```python
from build123d import *
from OCP.BRepFilletAPI import BRepFilletAPI_MakeChamfer

# Parameters (mm, degrees)
SKETCH1_W               = 29.5
SKETCH1_H               = 29.5
BOSS_EXTRUDE1_DEPTH     = 10
SKETCH2_R               = 12.5
CUT_EXTRUDE1_DEPTH      = 5
CHAMFER1_SIZE           = 22.860104606
CHAMFER1_SIZE_2         = 2
CHAMFER2_SIZE           = 4
CHAMFER2_SIZE2          = 4.030734246
SKETCH5_R               = 8
CUT_EXTRUDE2_DEPTH      = 10
BOSS_EXTRUDE2_START     = -1
BOSS_EXTRUDE2_DEPTH     = 1
MIRROR2_START           = -1
MIRROR2_COPY_1_DEPTH    = 1
CUT_EXTRUDE3_DEPTH      = 43.277768842
CUT_EXTRUDE3_DEPTH_BACK = 43.277768842
SKETCH7_R               = 1.125
SKETCH8_R               = 0.635
CUT_EXTRUDE4_DEPTH      = 43.501879232
SKETCH10_R              = 0.915
CUT_EXTRUDE5_DEPTH      = 2
SKETCH11_OUTSIDE_W      = 39.354
SKETCH11_OUTSIDE_H      = 39.324
SKETCH11_OUTSIDE_R      = 19
CUT_EXTRUDE6_DEPTH      = 43.501879232
SKETCH12_R              = 2
CUT_EXTRUDE7_DEPTH      = 9
SKETCH13_W              = 11
SKETCH13_H              = 30.855989766
CUT_EXTRUDE8_DEPTH      = 7


with BuildPart() as part:
    # Sketch1 → Boss-Extrude1 (new body)
    with BuildSketch(Plane(origin=(0, 0, 0), x_dir=(1, 0, 0), z_dir=(0, 1, 0))):
        with Locations((14.75, 14.75)):
            Rectangle(SKETCH1_W, SKETCH1_H)
    extrude(amount=BOSS_EXTRUDE1_DEPTH)

    # Sketch2 → Cut-Extrude1 (cut)
    with BuildSketch(Plane(origin=(0, 10, 0), x_dir=(1, 0, 0), z_dir=(0, 1, 0))):
        with Locations(Location((14.75, 14.75, 0), (0, 0, 270))):
            Circle(SKETCH2_R)
    extrude(amount=-CUT_EXTRUDE1_DEPTH, mode=Mode.SUBTRACT)

    # Chamfer1
    # the kernel refuses this chamfer: 22.860104606, 2 mm, written as the material it takes off along each edge
    with BuildSketch(Plane(origin=(-59.427907001, 0, 0), x_dir=(0, 1, 0), z_dir=(1, 0, 0)), Plane(origin=(29.5, 0, 59.427907001), x_dir=(0, 1, 0), z_dir=(0, 0, -1)), Plane(origin=(0, 0, -88.927907001), x_dir=(0, 1, 0), z_dir=(0, 0, 1))) as chamfer1_piece_1:
        Polygon((CHAMFER1_SIZE, 0), (0, -CHAMFER1_SIZE_2), (0, 0), align=None)
    extrude(amount=148.355814002, mode=Mode.SUBTRACT)
    with BuildSketch(Plane(origin=(88.927907001, 0, -29.5), x_dir=(0, 0, 1), z_dir=(-1, 0, 0))) as chamfer1_piece_2:
        Polygon((CHAMFER1_SIZE_2, 0), (0, CHAMFER1_SIZE), (0, 0), align=None)
    extrude(amount=148.355814002, mode=Mode.SUBTRACT)

    # Chamfer2: one chamfer whose edges measure the first distance from different faces: ONE call of the kernel's chamfer builder (chamfer() names one face for all edges)
    chamfer2_edges_1 = [part.edges().sort_by_distance(p)[0] for p in [
        (1.562556682, 5, -27.937443318),
        (27.937443318, 5, -27.937443318),
    ]]
    chamfer2_side_1 = [part.faces().sort_by_distance(p)[0] for p in [
        (14.75, 5.055285333, -27.942280158),
    ]]
    chamfer2_edges_2 = [part.edges().sort_by_distance(p)[0] for p in [
        (1.562556682, 5, -1.562556682),
    ]]
    chamfer2_side_2 = [part.faces().sort_by_distance(p)[0] for p in [
        (1.557719842, 5.055285333, -14.75),
    ]]
    chamfer2_edges_3 = [part.edges().sort_by_distance(p)[0] for p in [
        (27.937443318, 5, -1.562556682),
    ]]
    chamfer2_side_3 = [part.faces().sort_by_distance(p)[0] for p in [
        (27.942280158, 5.055285333, -14.75),
    ]]
    chamfer2 = BRepFilletAPI_MakeChamfer(part.part.solid().wrapped)
    for e in chamfer2_edges_1:
        chamfer2.Add(CHAMFER2_SIZE, CHAMFER2_SIZE2, e.wrapped, chamfer2_side_1[0].wrapped)  # the first distance lies on this face
    for e in chamfer2_edges_2:
        chamfer2.Add(CHAMFER2_SIZE, CHAMFER2_SIZE2, e.wrapped, chamfer2_side_2[0].wrapped)  # the first distance lies on this face
    for e in chamfer2_edges_3:
        chamfer2.Add(CHAMFER2_SIZE, CHAMFER2_SIZE2, e.wrapped, chamfer2_side_3[0].wrapped)  # the first distance lies on this face
    add(Compound.cast(chamfer2.Shape()), mode=Mode.REPLACE)

    # Sketch5 → Cut-Extrude2 (cut)
    with BuildSketch(Plane.XZ):
        with Locations(Location((14.75, -14.734574622, 0), (0, 0, 270))):
            Circle(SKETCH5_R)
    extrude(amount=-CUT_EXTRUDE2_DEPTH, mode=Mode.SUBTRACT)

    # Boss-Extrude2: read off the stored shape, not the designer's step
    # Boss-Extrude2 outline → Boss-Extrude2 (add)
    with BuildSketch(Plane(origin=(0, 10, 0), x_dir=(1, 0, 0), z_dir=(0, 1, 0)).offset(BOSS_EXTRUDE2_START)):
        with BuildLine():
            Line((1.125113365, 5.14027687), (5.171127626, 1.125113365))
            Line((5.171127626, 1.125113365), (24.328872374, 1.125113365))
            Line((24.328872374, 1.125113365), (28.374886635, 5.14027687))
            Line((28.374886635, 5.14027687), (28.374886635, 24.328872374))
            Line((28.374886635, 24.328872374), (24.35972313, 28.374886635))
            Line((24.35972313, 28.374886635), (5.14027687, 28.374886635))
            ThreePointArc((5.14027687, 28.374886635), (1.109687987, 28.359461258), (1.125113365, 24.328872374))
            Line((1.125113365, 24.328872374), (1.125113365, 5.14027687))
        make_face()
        Polygon((24.272234466, 28.287397972), (28.287397972, 24.241383711), (28.287397972, 5.227765534), (24.241383711, 1.212602028), (5.258616289, 1.212602028), (1.212602028, 5.227765534), (1.212602028, 24.241383711), (5.227765534, 28.287397972), align=None, mode=Mode.SUBTRACT)
    boss_extrude2 = extrude(amount=BOSS_EXTRUDE2_DEPTH)

    # Mirror1: Boss-Extrude2 across plane
    add(boss_extrude2.mirror(Plane(origin=(14.75, 0, 0), x_dir=(0, 0, 1), z_dir=(1, 0, 0))))

    # Mirror2: Boss-Extrude2 across plane
    add(boss_extrude2.mirror(Plane.XY.offset(-14.75)))

    # Mirror2 copy 1 sketch → Mirror2 copy 1 (add)
    with BuildSketch(Plane(origin=(29.5, 10, -29.5), x_dir=(-1, 0, 0), z_dir=(0, 1, 0)).offset(MIRROR2_START)):
        with BuildLine():
            Line((1.125113365, 5.14027687), (5.171127626, 1.125113365))
            Line((5.171127626, 1.125113365), (24.328872374, 1.125113365))
            Line((24.328872374, 1.125113365), (28.374886635, 5.14027687))
            Line((28.374886635, 5.14027687), (28.374886635, 24.328872374))
            Line((28.374886635, 24.328872374), (24.35972313, 28.374886635))
            Line((24.35972313, 28.374886635), (5.14027687, 28.374886635))
            ThreePointArc((5.14027687, 28.374886635), (1.109687987, 28.359461258), (1.125113365, 24.328872374))
            Line((1.125113365, 24.328872374), (1.125113365, 5.14027687))
        make_face()
        Polygon((24.272234466, 28.287397972), (28.287397972, 24.241383711), (28.287397972, 5.227765534), (24.241383711, 1.212602028), (5.258616289, 1.212602028), (1.212602028, 5.227765534), (1.212602028, 24.241383711), (5.227765534, 28.287397972), align=None, mode=Mode.SUBTRACT)
    extrude(amount=MIRROR2_COPY_1_DEPTH)

    # Sketch7 → Cut-Extrude3 (cut, two sides: drawn at the far end of the back side and taken through both)
    with BuildSketch(Plane.XZ.offset(-9).offset(-CUT_EXTRUDE3_DEPTH_BACK)):
        with Locations(Location((3.132695117, -3.148120495, 0), (0, 0, 270))):
            Circle(SKETCH7_R)
        with Locations(Location((26.367304883, -3.148120495, 0), (0, 0, 308.909428046))):
            Circle(SKETCH7_R)
        with Locations(Location((26.367304883, -26.351879505, 0), (0, 0, 270))):
            Circle(SKETCH7_R)
        with Locations(Location((3.132695117, -26.351879505, 0), (0, 0, 270))):
            Circle(SKETCH7_R)
    extrude(amount=CUT_EXTRUDE3_DEPTH + CUT_EXTRUDE3_DEPTH_BACK, mode=Mode.SUBTRACT)

    # Sketch8 → Cut-Extrude4 (cut, through all)
    with BuildSketch(Plane.XZ):
        with Locations(Location((7.375113365, -5.625113365, 0), (0, 0, 270))):
            Circle(SKETCH8_R)
        with Locations(Location((7.375113365, -23.874886635, 0), (0, 0, 270))):
            Circle(SKETCH8_R)
        with Locations(Location((4.625113365, -14.75, 0), (0, 0, 270))):
            Circle(SKETCH8_R)
        with Locations(Location((22.124886635, -23.874886635, 0), (0, 0, 90))):
            Circle(SKETCH8_R)
        with Locations(Location((24.874886635, -14.75, 0), (0, 0, 90))):
            Circle(SKETCH8_R)
        with Locations(Location((22.124886635, -5.625113365, 0), (0, 0, 90))):
            Circle(SKETCH8_R)
        with Locations(Location((5.770249527, -10.25, 0), (0, 0, 270))):
            Circle(SKETCH8_R)
        with Locations(Location((5.770249527, -19.25, 0), (0, 0, 90))):
            Circle(SKETCH8_R)
        with Locations(Location((23.729750473, -10.25, 0), (0, 0, 90))):
            Circle(SKETCH8_R)
        with Locations(Location((23.729750473, -19.25, 0), (0, 0, 270))):
            Circle(SKETCH8_R)
    extrude(amount=-CUT_EXTRUDE4_DEPTH, mode=Mode.SUBTRACT)

    # Sketch10 → Cut-Extrude5 (cut)
    with BuildSketch(Plane(origin=(0, 5, 0), x_dir=(1, 0, 0), z_dir=(0, 1, 0))):
        with Locations(Location((7.375113365, 23.874886635, 0), (0, 0, 270))):
            Circle(SKETCH10_R)
        with Locations(Location((4.625113365, 14.75, 0), (0, 0, 270))):
            Circle(SKETCH10_R)
        with Locations(Location((7.375113365, 5.625113365, 0), (0, 0, 270))):
            Circle(SKETCH10_R)
        with Locations(Location((22.124886635, 5.625113365, 0), (0, 0, 270))):
            Circle(SKETCH10_R)
        with Locations(Location((24.874886635, 14.75, 0), (0, 0, 270))):
            Circle(SKETCH10_R)
        with Locations(Location((22.124886635, 23.874886635, 0), (0, 0, 270))):
            Circle(SKETCH10_R)
        with Locations(Location((5.770249527, 19.25, 0), (0, 0, 270))):
            Circle(SKETCH10_R)
        with Locations(Location((5.770249527, 10.25, 0), (0, 0, 270))):
            Circle(SKETCH10_R)
        with Locations(Location((23.729750473, 10.25, 0), (0, 0, 270))):
            Circle(SKETCH10_R)
        with Locations(Location((23.729750473, 19.25, 0), (0, 0, 270))):
            Circle(SKETCH10_R)
    extrude(amount=-CUT_EXTRUDE5_DEPTH, mode=Mode.SUBTRACT)

    # Sketch11 outside → Cut-Extrude6 (cut, through all)
    with BuildSketch(Plane.XZ):
        with Locations((14.75, -14.75)):
            Rectangle(SKETCH11_OUTSIDE_W, SKETCH11_OUTSIDE_H)
        with Locations((14.75, -14.734574622)):
            Circle(SKETCH11_OUTSIDE_R, mode=Mode.SUBTRACT)
    extrude(amount=-CUT_EXTRUDE6_DEPTH, mode=Mode.SUBTRACT)

    # Sketch12 → Cut-Extrude7 (cut)
    with BuildSketch(Plane.XZ):
        with Locations((3.132695117, -3.148120495)):
            Circle(SKETCH12_R)
        with Locations((26.367304883, -3.148120495)):
            Circle(SKETCH12_R)
        with Locations((26.367304883, -26.351879505)):
            Circle(SKETCH12_R)
        with Locations((3.132695117, -26.351879505)):
            Circle(SKETCH12_R)
    extrude(amount=-CUT_EXTRUDE7_DEPTH, mode=Mode.SUBTRACT)

    # Sketch13 → Cut-Extrude8 (cut)
    with BuildSketch(Plane.XZ):
        with Locations((14.75, -15.427994883)):
            Rectangle(SKETCH13_W, SKETCH13_H)
    extrude(amount=-CUT_EXTRUDE8_DEPTH, mode=Mode.SUBTRACT)


solid = part.part
```
Geometry check sheet. Reference: the model listing, model coordinates, mm. A direction names the side the tool comes from. Give positions to 0.01 mm unless a question says otherwise; leave off trailing zeros. Order: outer loops, then holes, each group sorted by start corner. A loop starts at its lowest first (then second) coordinate and runs counter-clockwise, first axis right, second up. Notation, with made-up numbers: (-26, 57) - (17, 57) arc R35 ccw to (17, 96) - close; hole circle Ø7 at (-35, 48). An arc over 180 degrees is marked (long way). Write item = value, one per line. Start each with the question number.
1) Section check A-A (x = 14.75). Enter the section's corners in (y, z).
2) Section check B-B (y = 1). Count the separate pieces of the cut face and the enclosed holes in it, then the cut area to 3 significant figures.
3) Access from +Z, -Z, +X, -X, +Y, -Y to the whole of each face (thin tool, end or side, straight path). Record for faces 4 (the flat face through (25, 9, -4)), 5 (the flat face through (28.375, 9.5, -14.6)), 6 (the flat face through (14.7, 7, -27.5)), 7 (the flat face through (14.6, 9.5, -28.375)), 8 (the cylindrical face through (6.05, 4.01, -9.38)).
4) Section check D-D (y = 8.5). Enter the section's corners in (x, z).
5) Draft check along Z on faces 1 (the cylindrical face through (23.1, 1.48, -10.33)), 2 (the flat face through (9.25, 3, -24)), 3 (the flat face through (5.27, 4.44, -27.53)). Enter one of: released by +Z, released by -Z, zero draft, split by the parting line, or undercut.
6) Gauge pin test, flat ends, axial feed: pin 1 Ø0.5 at (x, z) = (24.5, -14.5) entering from +Y; pin 2 Ø2 at (y, z) = (2, -4.5) entering from +X; pin 3 Ø5 at (y, z) = (8, -9.5) entering from -X; pin 4 Ø1.5 at (x, z) = (22.12, -5.63) entering from -Y. Record the tip position at first contact, or that the pin passes through.
7) Scan lines: L1, parallel to Z at x = 6, y = 0.75; L2, parallel to Y at x = 25.75, z = -9.25; L3, parallel to X at y = 6.5, z = -7. Record each from-to range of solid material in increasing order.
Geometry check:
q1.outline = (7, -28.11) - (9, -28.29) - (9, -28.37) - (10, -28.37) - (10, -27.25) - (7, -27.25) - close; (7, -2.25) - (10, -2.25) - (10, -1.13) - (9, -1.13) - (9, -1.21) - (7, -1.39) - close
q2.separate_pieces = 2
q2.enclosed_holes = 10
q2.area = 283 mm2
q3.face_4 = -Y
q3.face_5 = +X, +Y, -Y
q3.face_6 = +Z, -Z, -Y
q3.face_7 = -Z, +Y, -Y
q3.face_8 = +Y
q4.outline = (1.26, -24.2) - (1.86, -24.81) arc R2 cw to (4.67, -27.63) - (5.27, -28.24) - (24.23, -28.24) - (24.83, -27.63) arc R2 cw to (27.64, -24.81) - (28.24, -24.2) - (28.24, -5.27) - (27.65, -4.68) arc R2 cw to (24.82, -1.88) - (24.2, -1.26) - (5.3, -1.26) - (4.68, -1.88) arc R2 cw to (1.85, -4.68) - (1.26, -5.27) - close; hole circle Ø25 at (14.75, -14.75)
q5.face_1 = undercut
q5.face_2 = zero draft
q5.face_3 = released by -Z
q6.pin_1 = 3
q6.pin_2 = 27.35
q6.pin_3 = 1.13
q6.pin_4 = 0
q7.L1 = -27.57 to -19.84, -18.66 to -10.84, -9.66 to -1.93
q7.L2 = 0 to 5
q7.L3 = 1.43 to 4.94, 24.56 to 28.07
